```python
from build123d import *

# Parameters (mm, degrees)
PAD_DEPTH = 203.2


with BuildPart() as part:
    # Sketch → Pad (new body)
    with BuildSketch(Plane.XZ):
        Polygon((-69.35, 0), (-69.35, 117), (-64.35, 117), (-64.35, 115), (-62.85, 115), (-62.85, 113), (-64.1, 113), (-64.1, 111), (-58.4, 111), (-58.4, 113), (-59.65, 113), (-59.65, 115), (-55.65, 115), (-55.65, 108.25), (-64.35, 99.55), (-64.35, 5), (0, 5), (0, 0), align=None)
    pad = extrude(amount=PAD_DEPTH)

    # Mirrored: Pad across Sketch V_Axis
    add(pad.mirror(Plane(origin=(0, 0, 0), x_dir=(0, -1, 0), z_dir=(1, 0, 0))))


solid = part.part
```
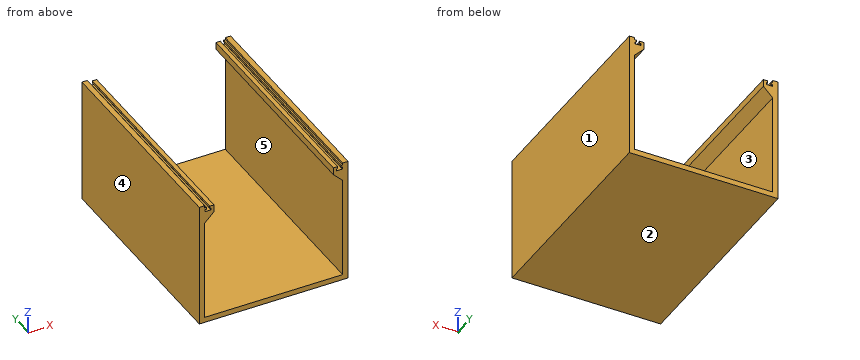
Design review of the part built by this model. Coordinates are the model's own, in mm. Face numbers are marked on the shaded views. A direction names the side the tool comes from. Round coordinates to 2 decimals unless told otherwise and drop trailing zeros. Write each loop counter-clockwise with the first axis right and the second up, starting at its lowest first coordinate (ties: lowest second). Pieces come first, ordered by that corner, then holes. Notation, with made-up numbers: (68, 79.25) -> (79, 79.25) arc R20 ccw to (79, 100.25) -> close; hole circle Ø1 at (-24, 67.25). An arc over 180 degrees is marked (long way). Write item = value, one per line. Start each with the question number.
1) Take a section at A-A, the plane z = 25.5. State the section outline as (x, y) points.
2) Take a section at C-C, the plane x = -48. State the section outline as (y, z) points, plus the area to 3 significant figures.
3) Wall thickness on probe 1 along X at (y, z) = (-151.5, 21.5); probe 2 along Z at (x, y) = (-5, -185.5); probe 3 along X at (y, z) = (-55, 103.5): over which ranges is each line inside the solid? List them lowest first. Write a range as from..to.
4) Mouldability with a two-part tool opening along X and no side actions: class the marked faces 1, 2 and 3 as +X half, -X half, draft (parallel to the pull), parting line (faces both ways), or undercut.
5) Clearance check with flat-ended pins moving along their axes: pin 1 (1.5 mm diameter, centred on x = 48.5, y = -100, fed in from +Z); pin 2 (3 mm diameter, centred on x = 60, y = -132, fed in from +Z). State where each tip first meets the part, or that it passes through.
6) Tool access review of the marked faces 4 and 5: name each direction out of +Z, -Z, +X, -X, +Y, -Y from which nothing blocks a thin tool from reaching the whole face with its end or side.
Results list:
q1.outline = (-69.35, -203.2) -> (-64.35, -203.2) -> (-64.35, 0) -> (-69.35, 0) -> close; (64.35, -203.2) -> (69.35, -203.2) -> (69.35, 0) -> (64.35, 0) -> close
q2.outline = (-203.2, 0) -> (0, 0) -> (0, 5) -> (-203.2, 5) -> close
q2.area = 1,020 mm²
q3.probe_1 = -69.35..-64.35, 64.35..69.35
q3.probe_2 = 0..5
q3.probe_3 = -69.35..-60.4, 60.4..69.35
q4.face_1 = +X half
q4.face_2 = draft
q4.face_3 = undercut
q5.pin_1 = 5
q5.pin_2 = 115
q6.face_4 = +Z, -Z, -X, +Y, -Y
q6.face_5 = +Y, -Y
